from build123d import *

# Parameters (mm, degrees)
SKETCH1_R                = 10
BOSS_EXTRUDE1_DEPTH      = 20
CUT_EXTRUDE10_DEPTH      = 12
CUT_EXTRUDE10_DEPTH_BACK = 12
CUT_SWEEP1_START         = -6.209273082
CUT_SWEEP1_OUTLINE_R     = 1.305
CUT_SWEEP1_DEPTH         = 3
CUT_SWEEP1_START_2       = 11.29177872
CUT_SWEEP1_2_OUTLINE_R   = 1.305
CUT_SWEEP1_2_DEPTH       = 8.70822128
CUT_SWEEP1_3_OUTLINE_R   = 1.305
CUT_SWEEP1_3_ANGLE       = 90
CUT_SWEEP2_START         = -11
CUT_SWEEP2_OUTLINE_R     = 2.5
CUT_SWEEP2_DEPTH         = 4.790726918
SKETCH25_W               = 5
SKETCH25_H               = 11.364916732
BOSS_EXTRUDE3_DEPTH      = 4.25
BOSS_EXTRUDE4_DEPTH      = 4.25
SKETCH27_R               = 0.935
CUT_EXTRUDE11_DEPTH      = 17.125
CUT_EXTRUDE12_START      = -0.75
CUT_EXTRUDE12_DEPTH      = 0.75
CUT_EXTRUDE13_DEPTH      = 10.375
SKETCH30_W               = 5
SKETCH30_H               = 4
CUT_EXTRUDE14_DEPTH      = 1.6
SCALE2_SCALE             = 0.8


with BuildPart() as part:
    # Sketch1 → Boss-Extrude1 (new body)
    with BuildSketch(Plane(origin=(0, 0, 0), x_dir=(0, 0, -1), z_dir=(1, 0, 0))):
        Circle(SKETCH1_R)
    extrude(amount=BOSS_EXTRUDE1_DEPTH)

    # Sketch12 → Revolve1 (revolve)
    with BuildSketch(Plane.XY):
        with BuildLine():
            Line((0, 10), (0, -10))
            ThreePointArc((0, -10), (-10, 0), (0, 10))
        make_face()
    revolve(axis=Axis((0, 10, 0), (0, -1, 0)))

    # Sketch13 → Cut-Extrude10 (cut, two sides: drawn at the far end of the back side and taken through both)
    with BuildSketch(Plane(origin=(0, 0, 0), x_dir=(1, 0, 0), z_dir=(0, 1, 0)).offset(-CUT_EXTRUDE10_DEPTH_BACK)):
        with BuildLine():
            ThreePointArc((-7.984675672, 6.020378262), (-3.764408562, -5.478068678), (7.618784032, -10))
            ThreePointArc((7.618784032, -10), (-7.804645707, -9.413161624), (-7.984675672, 6.020378262))
        make_face()
    extrude(amount=CUT_EXTRUDE10_DEPTH + CUT_EXTRUDE10_DEPTH_BACK, mode=Mode.SUBTRACT)

    # Cut-Sweep1: read off the stored shape, not the designer's step
    # Cut-Sweep1 outline → Cut-Sweep1 (cut)
    with BuildSketch(Plane.XY.offset(CUT_SWEEP1_START)):
        with Locations((1.29177882, 0)):
            Circle(CUT_SWEEP1_OUTLINE_R)
    extrude(amount=CUT_SWEEP1_DEPTH, mode=Mode.SUBTRACT)

    # Cut-Sweep1 2 outline → Cut-Sweep1 2 (cut)
    with BuildSketch(Plane.YZ.offset(CUT_SWEEP1_START_2)):
        with Locations((0, 6.790726918)):
            Circle(CUT_SWEEP1_2_OUTLINE_R)
    extrude(amount=CUT_SWEEP1_2_DEPTH, mode=Mode.SUBTRACT)

    # Cut-Sweep1 3 outline → Cut-Sweep1 3 (revolve, cut)
    with BuildSketch(Plane(origin=(11.29177882, 0, -3.209273082), x_dir=(-1, 0, 0), z_dir=(0, 0, -1))):
        with Locations((10, 0)):
            Circle(CUT_SWEEP1_3_OUTLINE_R)
    revolve(axis=Axis((11.29177882, 0, -3.209273082), (0, 1, 0)), revolution_arc=CUT_SWEEP1_3_ANGLE, mode=Mode.SUBTRACT)

    # Cut-Sweep2: read off the stored shape, not the designer's step
    # Cut-Sweep2 outline → Cut-Sweep2 (cut)
    with BuildSketch(Plane.XY.offset(CUT_SWEEP2_START)):
        with Locations((1.29177882, 0)):
            Circle(CUT_SWEEP2_OUTLINE_R)
    extrude(amount=CUT_SWEEP2_DEPTH, mode=Mode.SUBTRACT)

    # Sketch25 → Boss-Extrude3 (add)
    with BuildSketch(Plane(origin=(20, 0, 0), x_dir=(0, 0, -1), z_dir=(1, 0, 0))):
        Rectangle(SKETCH25_W, SKETCH25_H)
    extrude(amount=BOSS_EXTRUDE3_DEPTH)

    # Sketch26 → Boss-Extrude4 (add)
    with BuildSketch(Plane(origin=(20, 0, 0), x_dir=(0, 0, -1), z_dir=(1, 0, 0))):
        with BuildLine():
            Line((2.5, -9.682458366), (2.5, 9.682458366))
            ThreePointArc((2.5, 9.682458366), (10, 0), (2.5, -9.682458366))
        make_face()
    extrude(amount=BOSS_EXTRUDE4_DEPTH)

    # Sketch27 → Cut-Extrude11 (cut, symmetric)
    with BuildSketch(Plane(origin=(0, 0, 0), x_dir=(1, 0, 0), z_dir=(0, 1, 0))):
        with Locations(Location((22, 0.25, 0), (0, 0, 270))):
            Circle(SKETCH27_R)
    extrude(amount=CUT_EXTRUDE11_DEPTH, both=True, mode=Mode.SUBTRACT)

    # Sketch28 → Cut-Extrude12 (cut)
    with BuildSketch(Plane(origin=(20, 0, 0), x_dir=(0, 0, -1), z_dir=(1, 0, 0)).offset(CUT_EXTRUDE12_START)):
        with BuildLine():
            Line((2.5, -9.682458366), (2.5, -5.682458366))
            Line((2.5, -5.682458366), (-8.228588392, -5.682458366))
            ThreePointArc((-8.228588392, -5.682458366), (-3.493448331, -9.369942303), (2.5, -9.682458366))
        make_face()
        with BuildLine():
            Line((-8.228588392, 5.682458366), (2.5, 5.682458366))
            Line((2.5, 5.682458366), (2.5, 9.682458366))
            ThreePointArc((2.5, 9.682458366), (-3.493448331, 9.369942303), (-8.228588392, 5.682458366))
        make_face()
    extrude(amount=CUT_EXTRUDE12_DEPTH, mode=Mode.SUBTRACT)

    # Sketch29 → Cut-Extrude13 (cut, symmetric)
    with BuildSketch(Plane(origin=(0, 0, 0), x_dir=(1, 0, 0), z_dir=(0, 1, 0))):
        Polygon((20, -8.228588392), (20, -2.5), (12.5, -10), (20, -10), align=None)
    extrude(amount=CUT_EXTRUDE13_DEPTH, both=True, mode=Mode.SUBTRACT)

    # Sketch30 → Cut-Extrude14 (cut)
    with BuildSketch(Plane.XY.offset(-2.5)):
        with Locations((21.75, 7.682458366)):
            Rectangle(SKETCH30_W, SKETCH30_H)
        with Locations((21.75, -7.682458366)):
            Rectangle(SKETCH30_W, SKETCH30_H)
    extrude(amount=-CUT_EXTRUDE14_DEPTH, mode=Mode.SUBTRACT)


with BuildPart() as part_1:
    # Scale2: scaled about (8.050299805, 3.9953e-05, -0.823625188)
    add(part.part.scale(SCALE2_SCALE).moved(Location((1.610059961, 7.991e-06, -0.164725038))))


solid = part_1.part
Geometry check sheet. Reference: the model listing, model coordinates, mm. A direction names the side the tool comes from. Coordinates: 2 decimals unless noted, no trailing zeros. Order: outer loops, then holes, each group sorted by start corner. A loop starts at its lowest first (then second) coordinate and runs counter-clockwise, first axis right, second up. Notation, with made-up numbers: M 62.25,-10.75 L 94.25,-10.75 A33 ccw 94.25,24.25 Z; hole C -8.5,59.25 d1. An arc over 180 degrees is marked long. Use CSV: the item, a comma, the result in double quotes.
Item 1: Thickness scan on line 1 along Y through (x, z) = (0.75, 3); line 2 along X through (y, z) = (-0.25, -2); line 3 along X through (y, z) = (1.25, -5.5). Record the ranges inside material, lowest first.
Returned:
line 1,"y = -7.3 to 7.3"
line 2,"x = -4.61 to 1.66, 3.7 to 21.01"
line 3,"x = -4.22 to 1.08, 4.2 to 21.01"
Item 2: Cross-section at D-D on z = -0.75. Give the number of separate pieces and of enclosed holes in the cut face, then the cut area to 3 significant figures.
Returned:
separate pieces,"2"
enclosed holes,"1"
area,"352 mm2"
Item 3: Gauge pin test, flat ends, axial feed: pin 1 Ø1 at (y, z) = (-6, 0) entering from +X; pin 2 Ø4 at (x, y) = (5, 3) entering from +Z; pin 3 Ø3 at (x, z) = (15.5, -2) entering from -Y; pin 4 Ø4 at (y, z) = (6, 0.5) entering from +X. Record the tip position at first contact, or that the pin passes through.
Returned:
pin 1,"stops at x = 17.01"
pin 2,"stops at z = 7.75"
pin 3,"stops at y = -7.99"
pin 4,"stops at x = 21.01"
Item 4: Tool access check on faces 5 (the cylindrical face through (12.39, -0.23, 4.25)), 6 (the flat face through (18.5, -4.546, -1.1)), 7 (the flat face through (4, -1, -5.132)). Record the directions out of +Z, -Z, +X, -X, +Y, -Y that give a thin tool (end or side, any length) a straight path to the whole face; none if there is none.
Returned:
face 5,"+X"
face 6,"+Z, +X, -Y"
face 7,"-Z"
Item 5: Cross-section at A-A on y = -0.75. Record the cut outline in (x, z), then the cut area to 3 significant figures.
Returned:
outline,"M -4.78,-4.92 A7.96 ccw 0.79,-8.09 L 0.79,-5.13 L 1.92,-5.13 L 1.92,-2.73 A8.73 cw 10.64,5.99 L 13.45,5.99 L 11.65,7.8 L 6.15,7.8 A12 ccw Z; M 3.37,-5.13 L 4.5,-5.13 L 4.5,-8.13 L 21.01,-8.13 L 21.01,1.84 L 17.61,1.84 L 14.9,4.54 L 10.64,4.54 A7.27 ccw 3.37,-2.73 Z; hole C 19.21,-0.36 d1.5"
area,"297 mm2"
Item 6: Cross-section at B-B on z = -5.5. Record the cut outline in (x, y), then the cut area to 3 significant figures.
Returned:
outline,"M 1.61,-5.96 L 21.01,-5.96 L 21.01,5.96 L 1.61,5.96 A5.96 ccw Z; hole C 2.64,0 d4"
area,"275 mm2"
Item 7: Cross-section at C-C on y = -3. Record the cut outline in (x, z).
Returned:
outline,"M -4.8,-3.89 A7.42 ccw 1.61,-7.58 L 21.01,-7.58 L 21.01,1.84 L 17.61,1.84 L 12.19,7.25 L 3.47,7.25 A12 ccw Z; hole C 19.21,-0.36 d1.5"
Item 8: Mould release check, pull along Y, two halves, no side actions. Record for faces 1 (the cylindrical face through (18.48, 0.06, -0.53)), 2 (the cylindrical face through (0.645, 0.088, -6.67)), 3 (the cylindrical face through (9.02, 2.82, -7.65)), 4 (the cylindrical face through (1.6, 0, -3.9)): pulls with the +Y half, pulls with the -Y half, needs draft (parallel to the pull), parting line crosses it, or undercut.
Returned:
face 1,"needs draft"
face 2,"undercut"
face 3,"parting line crosses it"
face 4,"undercut"
